from build123d import *

# Parameters (mm, degrees)
BOSS_EXTRUDE1_DEPTH          = 60
CUT_EXTRUDE_THIN3_DEPTH      = 82.68933693
CUT_EXTRUDE_THIN3_DEPTH_BACK = 82.68933693
CUT_EXTRUDE_THIN4_DEPTH      = 82.68933693
CUT_EXTRUDE_THIN4_DEPTH_BACK = 82.68933693
BOSS_EXTRUDE4_DEPTH          = 10
BOSS_EXTRUDE5_DEPTH          = 10


with BuildPart() as part:
    # Sketch1 → Boss-Extrude1 (new body)
    with BuildSketch(Plane.XY):
        Polygon((-31.819805153, 31.819805153), (31.819805153, -31.819805153), (30.097767276, -33.541843031), (-33.541843031, 30.097767276), (-44.137201249, 30.097767276), (-44.137201249, 31.819805153), align=None)
    extrude(amount=BOSS_EXTRUDE1_DEPTH)

    # Sketch6 → Cut-Extrude-Thin3 (cut, two sides: drawn at the far end of the back side and taken through both)
    with BuildSketch(Plane(origin=(0, 0, 0), x_dir=(0.7071067811865561, -0.7071067811865389, 0), z_dir=(0.7071067811865389, 0.7071067811865561, 0)).offset(-CUT_EXTRUDE_THIN3_DEPTH_BACK)):
        Polygon((-45, -60), (45, -52.5774462), (86.096881173, -550.885630317), (-3.903118827, -558.308184117), align=None)
    extrude(amount=CUT_EXTRUDE_THIN3_DEPTH + CUT_EXTRUDE_THIN3_DEPTH_BACK, mode=Mode.SUBTRACT)

    # Sketch7 → Cut-Extrude-Thin4 (cut, two sides: drawn at the far end of the back side and taken through both)
    with BuildSketch(Plane(origin=(0, 0, 0), x_dir=(0.7071067811865561, -0.7071067811865389, 0), z_dir=(0.7071067811865389, 0.7071067811865561, 0)).offset(-CUT_EXTRUDE_THIN4_DEPTH_BACK)):
        Polygon((-45, 0), (45, -6.337900888), (80.123576931, 492.426907757), (-9.876423069, 498.764808646), align=None)
    extrude(amount=CUT_EXTRUDE_THIN4_DEPTH + CUT_EXTRUDE_THIN4_DEPTH_BACK, mode=Mode.SUBTRACT)

    # Sketch8 → Boss-Extrude4 (add)
    with BuildSketch(Plane(origin=(0, 0, 0), x_dir=(0, 0, -1), z_dir=(0.7071067811865389, 0.7071067811865561, 0))):
        Polygon((-60, 45), (-58.467214774, 45), (-51.473114592, -45), (-52.5774462, -45), align=None)
    extrude(amount=BOSS_EXTRUDE4_DEPTH)

    # Sketch9 → Boss-Extrude5 (add)
    with BuildSketch(Plane(origin=(0, 0, 0), x_dir=(0, 0, -1), z_dir=(0.7071067811865389, 0.7071067811865561, 0))):
        Polygon((-6.337900888, -45), (0, 45), (-1.653616098, 45), (-7.991516987, -45), align=None)
    extrude(amount=BOSS_EXTRUDE5_DEPTH)


solid = part.part
Read the model definition and answer for the solid it produces. Units are mm, in the model's axes. A direction names the side the tool comes from. Round coordinates to 2 decimals unless told otherwise and drop trailing zeros. Write each loop counter-clockwise with the first axis right and the second up, starting at its lowest first coordinate (ties: lowest second). Pieces come first, ordered by that corner, then holes. Notation, with made-up numbers: (74.25, 48) - (115.25, 48) arc R7 ccw to (115.25, 55) - close; hole circle Ø2 at (37, 48). An arc over 180 degrees is marked (long way). Use a Markdown table: item, result.
(1) Which of the six approach directions +Z, -Z, +X, -X, +Y, -Y give full straight-line access (tool end or side, diameter ignored) to faces 4 (the flat face through (3.04, 3.93, 4.78)), 5 (the flat face through (-39, 30.098, 30)), 6 (the flat face through (3.058, 2.167, 3.213))?
Reported:
| item | result |
|---|---|
| face 4 | +Y |
| face 5 | +Z, -Z, -X, -Y |
| face 6 | -Z, +X, -Y |
(2) The part is cut by section B-B (y = -22.5). Write down the section's boundary in (x, z).
Reported:
| item | result |
|---|---|
| outline | (19.06, 5.24) - (36.64, 6.11) - (36.64, 7.77) - (22.5, 7.06) - (22.5, 52.5) - (36.64, 51.72) - (36.64, 52.84) - (19.06, 53.87) - close |
(3) The mould has two halves that part along X. Classify faces 1 (the flat face through (3.04, 3.93, 55.02)), 2 (the flat face through (-28.33, 35.31, 0.82)), 3 (the flat face through (4.566, 9.577, 55.717)): released by +X, released by -X, zero draft, split by the parting line, or undercut.
Reported:
| item | result |
|---|---|
| face 1 | undercut |
| face 2 | released by -X |
| face 3 | released by +X |
(4) The part is cut by section C-C (x = -36). Write down the section's boundary in (y, z), then the cut area to 3 significant figures.
Reported:
| item | result |
|---|---|
| outline | (30.1, 0) - (31.82, 0) - (31.82, 60) - (30.1, 60) - close |
| area | 103 mm2 |
(5) The part is cut by section A-A (z = 46). Write down the section's boundary in (x, y), then the cut area to 3 significant figures.
Reported:
| item | result |
|---|---|
| outline | (-44.14, 30.1) - (-33.54, 30.1) - (30.1, -33.54) - (31.82, -31.82) - (-31.82, 31.82) - (-44.14, 31.82) - close |
| area | 239 mm2 |
(6) Straight lines are drawn through the part: line 1 along Z through (x, y) = (-5, 15); line 2 along X through (y, z) = (-24.5, 29); line 3 along Y through (x, z) = (-4, 5). For each, find the intervals that lie inside material, in ascending order. Write a range as [from, to].
Reported:
| item | result |
|---|---|
| line 1 | [2.17, 3.83], [56.07, 57.46] |
| line 2 | [21.06, 24.5] |
| line 3 | [0.56, 4] |
(7) The part is cut by section D-D (y = 33). Write down the section's boundary in (x, z), then the cut area to 3 significant figures.
Reported:
| item | result |
|---|---|
| outline | (-30.64, 0) - (-18.86, 0.59) - (-18.86, 2.24) - (-30.64, 1.65) - close; (-30.64, 58.47) - (-18.86, 57.82) - (-18.86, 59.31) - (-30.64, 60) - close |
| area | 37.3 mm2 |
(8) Each of these flat-tipped pins is pushed along its axis until it touches: pin 1 Ø3.5 at (x, z) = (-39.5, 24.5) entering from +Y; pin 2 Ø6 at (x, y) = (-10.5, 20) entering from +Z; pin 3 Ø2 at (x, z) = (-1.5, 52) entering from +Y. Where does it stop, or does it pass through?
Reported:
| item | result |
|---|---|
| pin 1 | y = 31.82 |
| pin 2 | z = 58.31 |
| pin 3 | y = 2.5 |
